Design review of the part built by this model. Coordinates are the model's own, in mm. Face numbers are marked on the shaded views. Give positions to 0.01 mm unless a question says otherwise; leave off trailing zeros. Write each loop counter-clockwise with the first axis right and the second up, starting at its lowest first coordinate (ties: lowest second). Pieces come first, ordered by that corner, then holes. Notation, with made-up numbers: (17, 64.5) - (55, 64.5) arc R15 cw to (55, 75.5) - close; hole circle Ø9 at (35.5, -1.75). An arc over 180 degrees is marked (long way). Use a Markdown table: item, result. Add a question column.
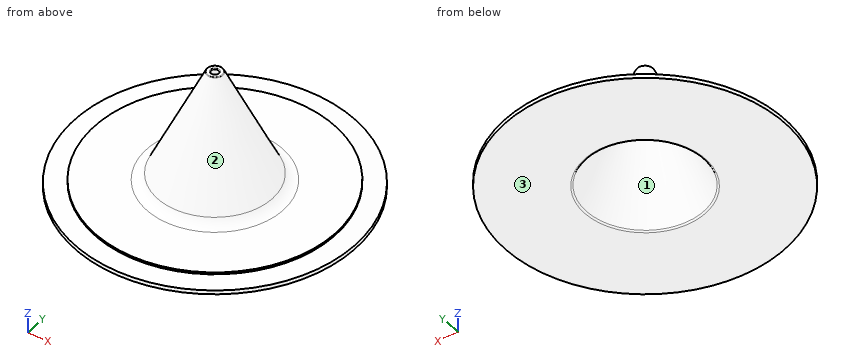
```python
from build123d import *

# Parameters (mm, degrees)
F2_R = 3


with BuildPart() as f1:
    # F0 (on Front) → F1 (revolve)
    with BuildSketch(Plane.XZ):
        with BuildLine():
            ThreePointArc((14.674281, 0.288557), (14.858785, 0.078265), (15.127373, 0))
            Line((15.127373, 0), (35, 0))
            Line((35, 0), (35, 1))
            Line((35, 1), (30, 1.173134))
            Line((30, 1.173134), (30, 1.673134))
            Line((30, 1.673134), (15.131675, 1.673134))
            Line((15.131675, 1.673134), (1.966335, 29.884577))
            ThreePointArc((1.966335, 29.884577), (1.892533, 29.968694), (1.785098, 30))
            Line((1.785098, 30), (1.12298, 30))
            ThreePointArc((1.12298, 30), (0.954286, 29.907435), (0.941744, 29.715423))
            Line((0.941744, 29.715423), (14.674281, 0.288557))
        make_face()
    revolve(axis=Axis((0, 0, 16.256472), (0, 0, 1)))

    # F2
    f2_edges = [f1.edges().sort_by_distance(p)[0] for p in [
        (-15.131675, 0, 1.673134),
    ]]
    fillet(f2_edges, radius=F2_R)


solid = f1.part
```
(1) For line 1 along X through (y, z) = (6.5, 14); line 2 along X through (y, z) = (-2.5, 14); line 3 along Y through (x, z) = (-1, 10), list the stretches that pass through material, from the lowest coordinate up.
(2) Add section C-C (z = 9). State the section outline as (x, y) points.
(3) Add section A-A (y = 0). State the section outline as (x, z) points.
(4) Insertion check: pin 1 (3 mm diameter, centred on x = -20.5, y = 5.5, fed in from +Z); pin 2 (1 mm diameter, centred on y = -7.5, z = 21.5, fed in from -X); pin 3 (12 mm diameter, centred on x = 2, z = 12.5, fed in from -Y); pin 4 (18 mm diameter, centred on x = 6, y = 13, fed in from +Z). Each pin has a flat end and moves straight along its axis. Give the tip position at first contact, or say it passes through.
(5) Add section D-D (z = 19.5). State the section outline as (x, y) points, and give its area (3 significant figures).
(6) Mouldability with a two-part tool opening along Y and no side actions: class the marked faces 1, 2 and 3 as +Y half, -Y half, draft (parallel to the pull), parting line (faces both ways), or undercut.
Answers follow:
| question | item | result |
|---|---|---|
| 1 | line 1 | -6.76 to -5.12, 5.12 to 6.76 |
| 1 | line 2 | -9.04 to -7.89, 7.89 to 9.04 |
| 1 | line 3 | -11.2 to -10.09, 10.09 to 11.2 |
| 2 | outline | circle Ø23.42 at (0, 0); hole circle Ø21.22 at (0, 0) |
| 3 | outline | (-35, 0) - (-15.13, 0) arc R0.5 ccw to (-14.67, 0.29) - (-0.94, 29.72) arc R0.2 ccw to (-1.12, 30) - (-1.79, 30) arc R0.2 ccw to (-1.97, 29.88) - (-14.32, 3.4) arc R3 cw to (-17.04, 1.67) - (-30, 1.67) - (-30, 1.17) - (-35, 1) - close; (0.94, 29.72) - (14.67, 0.29) arc R0.5 ccw to (15.13, 0) - (35, 0) - (35, 1) - (30, 1.17) - (30, 1.67) - (17.04, 1.67) arc R3 cw to (14.32, 3.4) - (1.97, 29.88) arc R0.2 ccw to (1.79, 30) - (1.12, 30) arc R0.2 ccw to start |
| 4 | pin 1 | z = 1.67 |
| 4 | pin 2 | through |
| 4 | pin 3 | y = -12.8 |
| 4 | pin 4 | z = 22.7 |
| 5 | outline | circle Ø13.62 at (0, 0); hole circle Ø11.42 at (0, 0) |
| 5 | area | 43.4 mm^2 |
| 6 | face 1 | undercut |
| 6 | face 2 | parting line |
| 6 | face 3 | draft |
